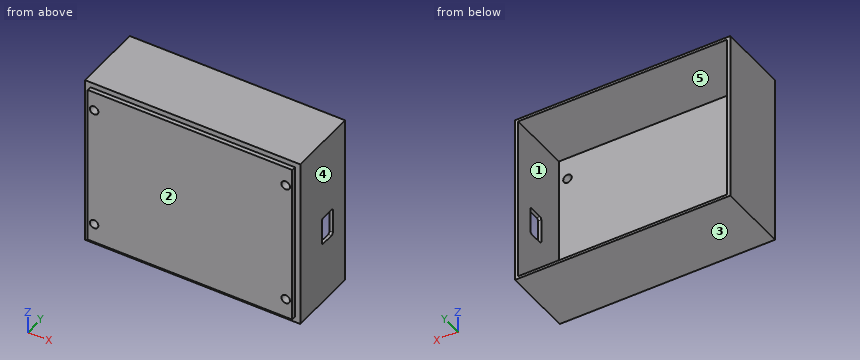
from build123d import *

# Parameters (mm, degrees)
SKETCH1_W           = 100
SKETCH1_H           = 80
BOSS_EXTRUDE1_DEPTH = 3
SKETCH2_W           = 100
SKETCH2_H           = 80
SKETCH2_W_2         = 97
SKETCH2_H_2         = 77.6
BOSS_EXTRUDE2_DEPTH = 30
SKETCH3_R           = 2
CUT_EXTRUDE1_DEPTH  = 40
SKETCH4_W           = 95
SKETCH4_H           = 75
BOSS_EXTRUDE3_DEPTH = 5
SKETCH3_2_R         = 2
CUT_EXTRUDE2_DEPTH  = 12
SKETCH5_W           = 13
SKETCH5_H           = 8
CUT_EXTRUDE3_DEPTH  = 10
FILLET1_R           = 1
FILLET2_R           = 1
FILLET3_R           = 1
FILLET4_R           = 1


with BuildPart() as part:
    # Sketch1 → Boss-Extrude1 (new body)
    with BuildSketch(Plane(origin=(0, 0, 0), x_dir=(1, 0, 0), z_dir=(0, 1, 0))):
        Rectangle(SKETCH1_W, SKETCH1_H)
    extrude(amount=BOSS_EXTRUDE1_DEPTH)

    # Sketch2 → Boss-Extrude2 (add)
    with BuildSketch(Plane(origin=(0, 3, 0), x_dir=(1, 0, 0), z_dir=(0, 1, 0))):
        Rectangle(SKETCH2_W, SKETCH2_H)
        Rectangle(SKETCH2_W_2, SKETCH2_H_2, mode=Mode.SUBTRACT)
    extrude(amount=BOSS_EXTRUDE2_DEPTH)

    # Sketch3 → Cut-Extrude1 (cut)
    with BuildSketch(Plane(origin=(0, 3, 0), x_dir=(1, 0, 0), z_dir=(0, 1, 0))):
        with Locations(Location((-44.5, 28.5, 0), (0, 0, 270))):
            Circle(SKETCH3_R)
        with Locations(Location((44.5, 28.5, 0), (0, 0, 270))):
            Circle(SKETCH3_R)
        with Locations(Location((-44.5, -28.5, 0), (0, 0, 270))):
            Circle(SKETCH3_R)
        with Locations(Location((44.5, -28.5, 0), (0, 0, 270))):
            Circle(SKETCH3_R)
    extrude(amount=-CUT_EXTRUDE1_DEPTH, mode=Mode.SUBTRACT)

    # Sketch4 → Boss-Extrude3 (add)
    with BuildSketch(Plane(origin=(0, 3, 0), x_dir=(1, 0, 0), z_dir=(0, 1, 0))):
        Rectangle(SKETCH4_W, SKETCH4_H)
    extrude(amount=-BOSS_EXTRUDE3_DEPTH)

    # Sketch3_2 → Cut-Extrude2 (cut)
    with BuildSketch(Plane(origin=(0, 3, 0), x_dir=(1, 0, 0), z_dir=(0, 1, 0))):
        with Locations(Location((-44.5, 28.5, 0), (0, 0, 270))):
            Circle(SKETCH3_2_R)
        with Locations(Location((44.5, 28.5, 0), (0, 0, 270))):
            Circle(SKETCH3_2_R)
        with Locations(Location((-44.5, -28.5, 0), (0, 0, 270))):
            Circle(SKETCH3_2_R)
        with Locations(Location((44.5, -28.5, 0), (0, 0, 270))):
            Circle(SKETCH3_2_R)
    extrude(amount=-CUT_EXTRUDE2_DEPTH, mode=Mode.SUBTRACT)

    # Sketch5 → Cut-Extrude3 (cut)
    with BuildSketch(Plane(origin=(50, 0, 0), x_dir=(0, 0, -1), z_dir=(1, 0, 0))):
        with Locations((4.6, 20)):
            Rectangle(SKETCH5_W, SKETCH5_H)
    extrude(amount=-CUT_EXTRUDE3_DEPTH, mode=Mode.SUBTRACT)

    # Fillet1
    fillet1_edges = [part.edges().sort_by_distance(p)[0] for p in [
        (49.25, 24, -11.1),
    ]]
    fillet(fillet1_edges, radius=FILLET1_R)

    # Fillet2
    fillet2_edges = [part.edges().sort_by_distance(p)[0] for p in [
        (49.25, 24, 1.9),
    ]]
    fillet(fillet2_edges, radius=FILLET2_R)

    # Fillet3
    fillet3_edges = [part.edges().sort_by_distance(p)[0] for p in [
        (49.25, 16, 1.9),
    ]]
    fillet(fillet3_edges, radius=FILLET3_R)

    # Fillet4
    fillet4_edges = [part.edges().sort_by_distance(p)[0] for p in [
        (49.25, 16, -11.1),
    ]]
    fillet(fillet4_edges, radius=FILLET4_R)


solid = part.part
Verification items for the finished model (mm, model axes). Face numbers are marked on the shaded views. A direction names the side the tool comes from. Round coordinates to 2 decimals unless told otherwise and drop trailing zeros. Loops run counter-clockwise (first coordinate to the right, second up) from the corner with the lowest first, then second, coordinate; pieces in that order, holes last. Notation, with made-up numbers: M -0.5,-17.5 L 56.5,-17.5 A22 ccw 56.5,-5.5 Z; hole C 58.25,-6.75 d3. An arc over 180 degrees is marked long. Write each question's results on one line, items separated by ' | '.
1) Gauge pin test, flat ends, axial feed: P1, Ø1, axis at x = -9.5, y = -1, coming from the +Z side; P2, Ø8, axis at x = -39.5, z = 3.5, coming from the +Y side; P3, Ø3, axis at x = -44.5, z = 28.5, coming from the +Y side; P4, Ø0.6, axis at x = 2.5, y = -1, coming from the -Z side. Record the tip position at first contact, or that the pin passes through.
Checks:
P1: stops at z = 37.5 | P2: stops at y = 3 | P3: passes through | P4: stops at z = -37.5
2) Access from +Z, -Z, +X, -X, +Y, -Y to the whole of each face (thin tool, end or side, straight path). Record for the marked faces 4 and 5.
Checks:
face 4: +Z, -Z, +X, +Y, -Y | face 5: +Y
3) Section check D-D on z = -28.5. Record the boundary of the cut face in (x, y).
Checks:
outline: M -50,0 L -47.5,0 L -47.5,-2 L -46.5,-2 L -46.5,3 L -48.5,3 L -48.5,33 L -50,33 Z; M -42.5,-2 L 42.5,-2 L 42.5,3 L -42.5,3 Z; M 46.5,-2 L 47.5,-2 L 47.5,0 L 50,0 L 50,33 L 48.5,33 L 48.5,3 L 46.5,3 Z
4) Section check B-B on z = -3. Record the boundary of the cut face in (x, y).
Checks:
outline: M -50,0 L -47.5,0 L -47.5,-2 L 47.5,-2 L 47.5,0 L 50,0 L 50,16 L 48.5,16 L 48.5,3 L -48.5,3 L -48.5,33 L -50,33 Z; M 48.5,24 L 50,24 L 50,33 L 48.5,33 Z
5) Mould release check, pull along Z, two halves, no side actions. Record for the marked faces 1, 2 and 3: released by +Z, released by -Z, zero draft, split by the parting line, or undercut.
Checks:
face 1: undercut | face 2: zero draft | face 3: released by -Z
6) Scan lines: L1, parallel to X at y = -0.95, z = 28.5; L2, parallel to Z at x = 6.5, y = 11; L3, parallel to X at y = 0.75, z = 28.5. Record each from-to range of solid material in increasing order. Write a range as from..to.
Checks:
L1: x = -47.5..-46.5, -42.5..42.5, 46.5..47.5 | L2: z = -40..-38.8, 38.8..40 | L3: x = -50..-46.5, -42.5..42.5, 46.5..50
7) Section check A-A on y = 27. Record the boundary of the cut face in (x, z).
Checks:
outline: M -50,-40 L 50,-40 L 50,40 L -50,40 Z; hole M -48.5,-38.8 L 48.5,-38.8 L 48.5,38.8 L -48.5,38.8 Z
8) Section check C-C on x = 44.5. Record the boundary of the cut face in (y, z).
Checks:
outline: M -2,-37.5 L 0,-37.5 L 0,-40 L 33,-40 L 33,-38.8 L 3,-38.8 L 3,-30.5 L -2,-30.5 Z; M -2,-26.5 L 3,-26.5 L 3,26.5 L -2,26.5 Z; M -2,30.5 L 3,30.5 L 3,38.8 L 33,38.8 L 33,40 L 0,40 L 0,37.5 L -2,37.5 Z
